The model under review builds one solid part; all positions refer to its coordinate system, in mm. Face numbers are marked on the shaded views. A direction names the side the tool comes from. Coordinates: 2 decimals unless noted, no trailing zeros. Order: outer loops, then holes, each group sorted by start corner. A loop starts at its lowest first (then second) coordinate and runs counter-clockwise, first axis right, second up. Notation, with made-up numbers: M -5,1 L 1,1 A22 cw 1,10 Z; hole C -38,45.25 d6. An arc over 180 degrees is marked long. Answer as CSV lines item,"result". Start each with the question number.
Q1. Consider section B-B on z = -27. Write out the cut boundary in (x, y) (3 decimals).
Q2. Machinability: for the marked faces 1, 2, 3 and 4, which of the approach directions +Z, -Z, +X, -X, +Y, -Y give a long, thin tool a straight path to every point of the face, cutting with its end or side? Answer none if there is none.
Q3. Consider section D-D on x = 11.5. Write out the cut boundary in (y, z) (1 decimal), and give its area (3 significant figures).
Q4. For P1, Ø2, axis at x = 13, z = -14.5, coming from the +Y side (3 decimals); P2, Ø5, axis at x = 7.62, z = -34.41, coming from the -Y side; P3, Ø2, axis at x = 10, z = 2, coming from the -Y side; P4, Ø4, axis at x = 9, z = -28.5, coming from the -Y side, all flat-tipped, find the tip position at first contact; note any pin that passes through.
Q5. The part is to be moulded in two halves that separate along Y. For the marked faces 5, 6, 7 and 8, say which applies: +Y half, -Y half, draft (parallel to the pull), parting line (faces both ways), or undercut.
Q6. Wall thickness on L1, parallel to Z at x = 7.62, y = 24.25; L2, parallel to Y at x = 3.75, z = -18.5 (3 decimals); L3, parallel to Y at x = 6, z = 4: over which ranges is each line inside the solid? List them lowest first. Write a range as [from, to].
Q7. Consider section A-A on x = 7.62. State how many separate pieces and enclosed holes the cut face has, and give its area (3 significant figures).
Q8. Consider section C-C on y = 26.5. Write out the cut boundary in (x, z), and give its area (3 significant figures).
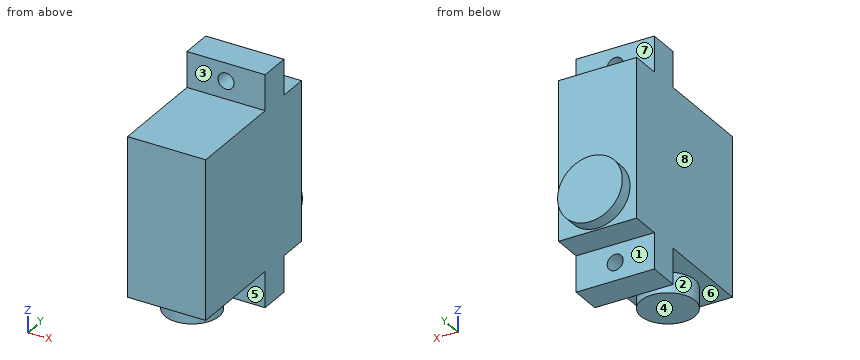
from build123d import *

# Parameters (mm, degrees)
SKETCH1_W                = 15.24
SKETCH1_H                = 30.9118
BOSS_EXTRUDE1_DEPTH      = 31.115
SKETCH2_W                = 15.24
SKETCH2_H                = 6.096
BOSS_EXTRUDE2_DEPTH      = 6.9215
BOSS_EXTRUDE2_DEPTH_BACK = 37.9095
SKETCH3_R                = 5.2705
BOSS_EXTRUDE3_DEPTH      = 3.9624
SKETCH4_R                = 6.3119
BOSS_EXTRUDE4_DEPTH      = 2.5019
CUT_EXTRUDE1_REACH       = 27.4
SKETCH8_R                = 1.5621
CUT_EXTRUDE2_REACH       = 27.4
SKETCH9_R                = 1.5621


with BuildPart() as part:
    # Sketch1 → Boss-Extrude1 (new body)
    with BuildSketch(Plane(origin=(0, 0, 0), x_dir=(1, 0, 0), z_dir=(0, 1, 0))):
        with Locations((7.62, 15.4559)):
            Rectangle(SKETCH1_W, SKETCH1_H)
    extrude(amount=BOSS_EXTRUDE1_DEPTH)

    # Sketch2 → Boss-Extrude2 (add, two sides)
    with BuildSketch(Plane.XY) as boss_extrude2_sk:
        with Locations((7.62, 22.352)):
            Rectangle(SKETCH2_W, SKETCH2_H)
    extrude(amount=BOSS_EXTRUDE2_DEPTH)
    extrude(boss_extrude2_sk.sketch, amount=-BOSS_EXTRUDE2_DEPTH_BACK)

    # Sketch3 → Boss-Extrude3 (add)
    with BuildSketch(Plane(origin=(0, 0, -30.9118), x_dir=(-1, 0, 0), z_dir=(0, 0, -1))):
        with Locations((-7.62, 8.2804)):
            Circle(SKETCH3_R)
    extrude(amount=BOSS_EXTRUDE3_DEPTH)

    # Sketch4 → Boss-Extrude4 (add)
    with BuildSketch(Plane(origin=(0, 31.115, 0), x_dir=(1, 0, 0), z_dir=(0, 1, 0))):
        with Locations((7.62, 24.2951)):
            Circle(SKETCH4_R)
    extrude(amount=BOSS_EXTRUDE4_DEPTH)

    # Sketch8 → Cut-Extrude1 (cut, up to next)
    with BuildSketch(Plane(origin=(0, 25.4, 0), x_dir=(1, 0, 0), z_dir=(0, 1, 0)), mode=Mode.PRIVATE) as cut_extrude1_sk1:
        with Locations((7.62, -3.46075)):
            Circle(SKETCH8_R)
    cut_extrude1_tool1 = extrude(cut_extrude1_sk1.sketch, amount=-CUT_EXTRUDE1_REACH, mode=Mode.PRIVATE) & part.part
    add(cut_extrude1_tool1.solids().sort_by_distance((7.62, 25.4, 3.46075))[0], mode=Mode.SUBTRACT)

    # Sketch9 → Cut-Extrude2 (cut, up to next)
    with BuildSketch(Plane(origin=(0, 25.4, 0), x_dir=(1, 0, 0), z_dir=(0, 1, 0)), mode=Mode.PRIVATE) as cut_extrude2_sk1:
        with Locations((7.62, 34.41065)):
            Circle(SKETCH9_R)
    cut_extrude2_tool1 = extrude(cut_extrude2_sk1.sketch, amount=-CUT_EXTRUDE2_REACH, mode=Mode.PRIVATE) & part.part
    add(cut_extrude2_tool1.solids().sort_by_distance((7.62, 25.4, -34.41065))[0], mode=Mode.SUBTRACT)


solid = part.part
Evaluation:
1,outline,"M 0,0 L 15.24,0 L 15.24,31.115 L 13.323,31.115 L 13.323,33.617 L 1.917,33.617 L 1.917,31.115 L 0,31.115 Z"
2,face 1,"-Z, +X, -X, +Y"
2,face 2,"-Z"
2,face 3,"+Z, +X, -X, -Y"
2,face 4,"-Z, +X, -X, -Y"
3,outline,"M 0,-30.9 L 4.7,-30.9 L 4.7,-34.9 L 11.8,-34.9 L 11.8,-30.9 L 19.3,-30.9 L 19.3,-37.9 L 25.4,-37.9 L 25.4,-30.9 L 31.1,-30.9 L 31.1,-29.3 L 33.6,-29.3 L 33.6,-19.3 L 31.1,-19.3 L 31.1,0 L 25.4,0 L 25.4,6.9 L 19.3,6.9 L 19.3,0 L 0,0 Z"
3,area,"1,100 mm²"
4,P1,"stops at y = 31.115"
4,P2,"stops at y = 3.01"
4,P3,"stops at y = 19.3"
4,P4,"stops at y = 0"
5,face 5,"undercut"
5,face 6,"undercut"
5,face 7,"+Y half"
5,face 8,"draft"
6,L1,"z = [-37.91, -35.97], [-32.85, 1.9], [5.02, 6.92]"
6,L2,"y = [0, 31.115]"
6,L3,"y = [19.3, 25.4]"
7,separate pieces,"3"
7,enclosed holes,"0"
7,area,"1,080 mm²"
8,outline,"M 0,-30.91 L 15.24,-30.91 L 15.24,0 L 0,0 Z"
8,area,"471 mm²"
